from build123d import *

# Parameters (mm, degrees)
F0_W     = 210
F0_H     = 201
F1_DEPTH = 3
F2_W     = 72
F2_H     = 135
F3_DEPTH = 3.001
F4_R     = 5
F5_R     = 3.5
F5_R_2   = 5.1
F6_DEPTH = 3.001
F7_R     = 8.5
F8_DEPTH = 1.5


with BuildPart() as f1:
    # F0 (on Top) → F1 (new body)
    with BuildSketch(Plane.XY):
        Rectangle(F0_W, F0_H)
    extrude(amount=-F1_DEPTH)

    # F2 (on face) → F3 (cut, through all)
    with BuildSketch(Plane.XY):
        with Locations((69, -33)):
            Rectangle(F2_W, F2_H)
        with Locations((-69, -33)):
            Rectangle(F2_W, F2_H)
    extrude(amount=-F3_DEPTH, mode=Mode.SUBTRACT)

    # F4
    f4_edges = [f1.edges().sort_by_distance(p)[0] for p in [
        (33, -100.5, -1.5),
        (33, 34.5, -1.5),
        (105, 34.5, -1.5),
        (105, 100.5, -1.5),
        (-33, -100.5, -1.5),
        (-33, 34.5, -1.5),
        (-105, 34.5, -1.5),
        (-105, 100.5, -1.5),
    ]]
    fillet(f4_edges, radius=F4_R)

    # F5 (on face) → F6 (cut, through all)
    with BuildSketch(Plane.XY):
        with Locations((-90, 87.5)):
            Circle(F5_R)
        with Locations((-90, 47.5)):
            Circle(F5_R)
        with Locations((-50, 87.5)):
            Circle(F5_R)
        with Locations((-50, 47.5)):
            Circle(F5_R)
        with Locations((-70, 67.5)):
            Circle(F5_R_2)
        with Locations((-20, 87.5)):
            Circle(F5_R)
        with Locations((20, 87.5)):
            Circle(F5_R)
        with Locations((50, 87.5)):
            Circle(F5_R)
        with Locations((90, 87.5)):
            Circle(F5_R)
        with Locations((-20, 47.5)):
            Circle(F5_R)
        with Locations((20, 47.5)):
            Circle(F5_R)
        with Locations((50, 47.5)):
            Circle(F5_R)
        with Locations((90, 47.5)):
            Circle(F5_R)
        with Locations((-35, 67.5)):
            Circle(F5_R_2)
        with Locations((0, 67.5)):
            Circle(F5_R_2)
        with Locations((35, 67.5)):
            Circle(F5_R_2)
        with Locations((70, 67.5)):
            Circle(F5_R_2)
        with Locations((-20, 17.5)):
            Circle(F5_R)
        with Locations((-20, -92.5)):
            Circle(F5_R)
        with BuildLine():
            ThreePointArc((-16.5, -17.5), (-20, -14), (-23.5, -17.5))
            Line((-23.5, -17.5), (-23.5, -22.5))
            ThreePointArc((-23.5, -22.5), (-20, -26), (-16.5, -22.5))
            Line((-16.5, -22.5), (-16.5, -17.5))
        make_face()
        with BuildLine():
            ThreePointArc((-16.5, -52.5), (-20, -49), (-23.5, -52.5))
            Line((-23.5, -52.5), (-23.5, -57.5))
            ThreePointArc((-23.5, -57.5), (-20, -61), (-16.5, -57.5))
            Line((-16.5, -57.5), (-16.5, -52.5))
        make_face()
        with Locations((20, -92.5)):
            Circle(F5_R)
        with BuildLine():
            Line((16.5, -52.5), (16.5, -57.5))
            ThreePointArc((16.5, -57.5), (20, -61), (23.5, -57.5))
            Line((23.5, -57.5), (23.5, -52.5))
            ThreePointArc((23.5, -52.5), (20, -49), (16.5, -52.5))
        make_face()
        with BuildLine():
            Line((23.5, -22.5), (23.5, -17.5))
            ThreePointArc((23.5, -17.5), (20, -14), (16.5, -17.5))
            Line((16.5, -17.5), (16.5, -22.5))
            ThreePointArc((16.5, -22.5), (20, -26), (23.5, -22.5))
        make_face()
        with Locations((20, 17.5)):
            Circle(F5_R)
        with Locations((0, -2.5)):
            Circle(F5_R_2)
        with Locations((0, -37.5)):
            Circle(F5_R_2)
        with Locations((0, -72.5)):
            Circle(F5_R_2)
    extrude(amount=-F6_DEPTH, mode=Mode.SUBTRACT)

    # F7 (on face) → F8 (cut)
    with BuildSketch(Plane.XY):
        with Locations((-70, 67.5)):
            Circle(F7_R)
        with Locations((-35, 67.5)):
            Circle(F7_R)
        with Locations((0, 67.5)):
            Circle(F7_R)
        with Locations((35, 67.5)):
            Circle(F7_R)
        with Locations((70, 67.5)):
            Circle(F7_R)
        with Locations((0, -72.5)):
            Circle(F7_R)
        with Locations((0, -37.5)):
            Circle(F7_R)
        with Locations((0, -2.5)):
            Circle(F7_R)
    extrude(amount=-F8_DEPTH, mode=Mode.SUBTRACT)


solid = f1.part
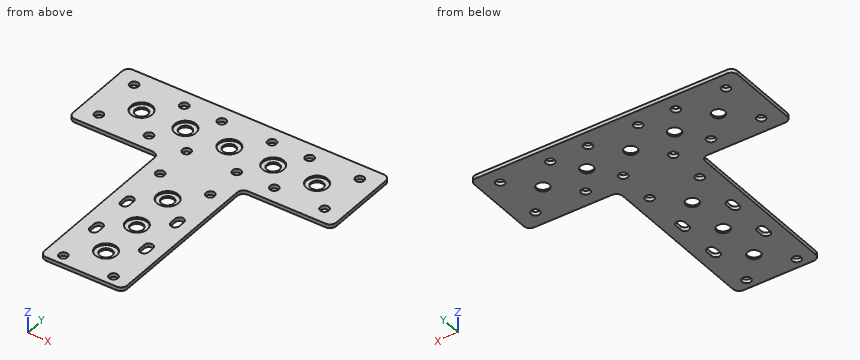
Geometry check sheet. Reference: the model listing, model coordinates, mm. Round coordinates to 2 decimals unless told otherwise and drop trailing zeros. Write each loop counter-clockwise with the first axis right and the second up, starting at its lowest first coordinate (ties: lowest second). Pieces come first, ordered by that corner, then holes. Notation, with made-up numbers: (87, -26.75) -> (133, -26.75) arc R9 cw to (133, -19.75) -> close; hole circle Ø1 at (-27, 66). An arc over 180 degrees is marked (long way). One line per item, written item: value. Start each with the question number.
(1) Cross-section at C-C, the plane y = -37.5. Record the cut outline in (x, z).
(2) Cross-section at A-A, the plane x = 70. Record the cut outline in (y, z), and give its area (3 significant figures).
(3) Go/stop test with flat-tipped pins: pin 1 Ø5 at (x, y) = (72.5, 67) entering from +Z; pin 2 Ø1 at (x, z) = (62.5, -1.5) entering from -Y; pin 3 Ø1.5 at (y, z) = (-19.5, -1.5) entering from -X. Record where each tip stops, or that it passes through.
(4) Cross-section at D-D, the plane z = -0.9. Give the number of separate pieces and of enclosed holes in the cut face, and give its area (3 significant figures).
(5) Cross-section at B-B, the plane y = 47.5. Record the cut outline in (x, z), and give its area (3 significant figures).
(6) Scan lines: line 1 (X direction, y = 17, z = -0.35); line 2 (Y direction, x = -90, z = -1.5); line 3 (X direction, y = 16.5, z = -2.1). Record each from-to range of solid material in increasing order. Write a range as [from, to].
Answer:
1. outline: (-33, -3) -> (-5.1, -3) -> (-5.1, -1.5) -> (-8.5, -1.5) -> (-8.5, 0) -> (-33, 0) -> close; (5.1, -3) -> (33, -3) -> (33, 0) -> (8.5, 0) -> (8.5, -1.5) -> (5.1, -1.5) -> close
2. outline: (34.5, -3) -> (62.4, -3) -> (62.4, -1.5) -> (59, -1.5) -> (59, 0) -> (34.5, 0) -> close; (72.6, -3) -> (100.5, -3) -> (100.5, 0) -> (76, 0) -> (76, -1.5) -> (72.6, -1.5) -> close
2. area: 157 mm²
3. pin 1: through
3. pin 2: y = 34.5
3. pin 3: x = -33
4. separate pieces: 1
4. enclosed holes: 28
4. area: 20,000 mm²
5. outline: (-105, -3) -> (-93.5, -3) -> (-93.5, 0) -> (-105, 0) -> close; (-86.5, -3) -> (-53.5, -3) -> (-53.5, 0) -> (-86.5, 0) -> close; (-46.5, -3) -> (-23.5, -3) -> (-23.5, 0) -> (-46.5, 0) -> close; (-16.5, -3) -> (16.5, -3) -> (16.5, 0) -> (-16.5, 0) -> close; (23.5, -3) -> (46.5, -3) -> (46.5, 0) -> (23.5, 0) -> close; (53.5, -3) -> (86.5, -3) -> (86.5, 0) -> (53.5, 0) -> close; (93.5, -3) -> (105, -3) -> (105, 0) -> (93.5, 0) -> close
5. area: 504 mm²
6. line 1: [-33, -23.46], [-16.54, 16.54], [23.46, 33]
6. line 2: [34.5, 44], [51, 84], [91, 100.5]
6. line 3: [-33, -23.35], [-16.65, 16.65], [23.35, 33]
